The drawing under review shows one solid part. Ordinate dimensions are in mm from its lowest x, y, z. A direction names the side the tool comes from. Round coordinates to 2 decimals unless told otherwise and drop trailing zeros. Loops run counter-clockwise (first coordinate to the right, second up) from the corner with the lowest first, then second, coordinate; pieces in that order, holes last. Notation, with made-up numbers: (61, 44.5) - (91, 44.5) arc R16 ccw to (91, 67.5) - close; hole circle Ø11 at (-38, 11). An arc over 180 degrees is marked (long way). Answer as CSV lines item,"result".
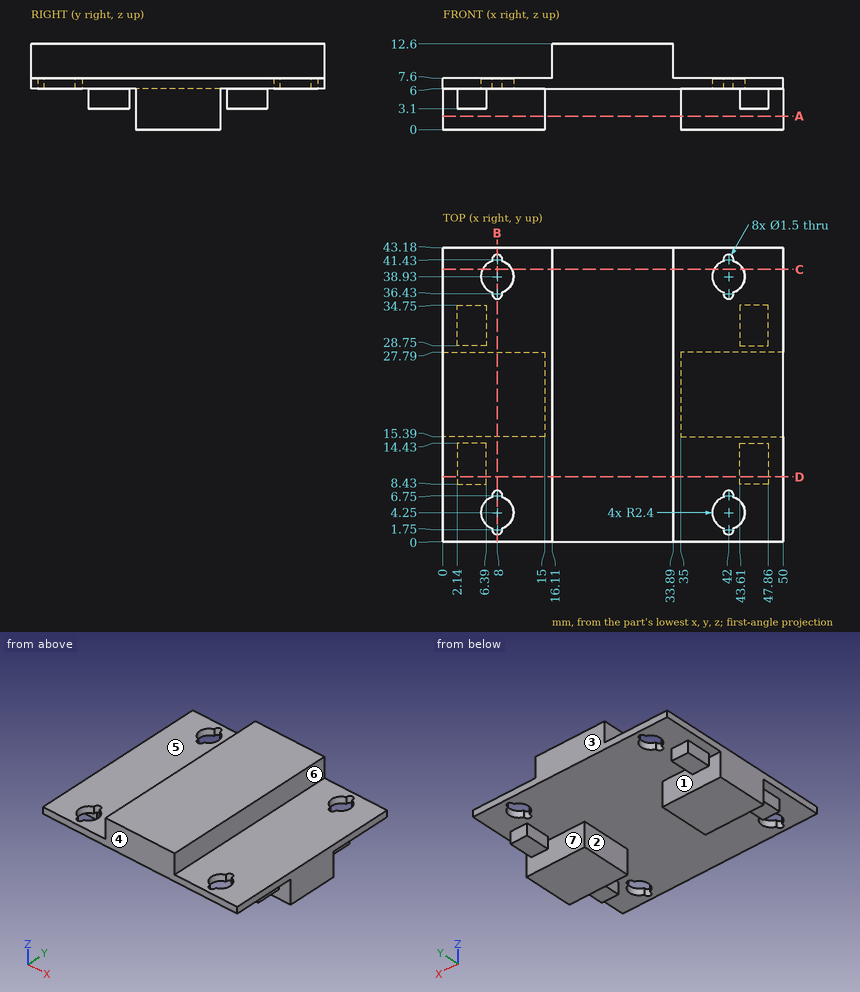
1. Take a section at B-B (x = 8). State the section outline as (y, z) points, plus the area to 3 significant figures.
Numbers:
outline,"(0, 6) - (1, 6) - (1, 7.6) - (0, 7.6) - close; (7.5, 6) - (15.39, 6) - (15.39, 0) - (27.79, 0) - (27.79, 6) - (35.68, 6) - (35.68, 7.6) - (7.5, 7.6) - close; (42.18, 6) - (43.18, 6) - (43.18, 7.6) - (42.18, 7.6) - close"
area,"123 mm²"
2. Wall thickness on probe 1 along X at (y, z) = (6.75, 6.5); probe 2 along X at (y, z) = (23, 3.5); probe 3 along Z at (x, y) = (17.5, 36.5): over which ranges is each line inside the solid? List them lowest first.
Numbers:
probe 1,"x = 0 to 7.25, 8.75 to 41.25, 42.75 to 50"
probe 2,"x = 0 to 15, 35 to 50"
probe 3,"z = 6 to 12.6"
3. Clearance check with flat-ended pins moving along their axes: pin 1 (0.9 mm diameter, centred on y = 32, z = 4.5, fed in from -X); pin 2 (4.5 mm diameter, centred on x = 45, y = 32, fed in from -Z); pin 3 (8 mm diameter, centred on x = 34.5, y = 8.5, fed in from -Z); pin 4 (3 mm diameter, centred on x = 29, z = 5.5, fed in from -Y). State where each tip first meets the part, or that it passes through.
Numbers:
pin 1,"stops at x = 2.14"
pin 2,"stops at z = 3.1"
pin 3,"stops at z = 6"
pin 4,"stops at y = 0"
4. Draft analysis for pull direction Y (two halves, no side actions). For the marked faces 1, 2, 3 and 4, state which applies: +Y half, -Y half, draft (parallel to the pull), parting line (faces both ways), or undercut.
Numbers:
face 1,"undercut"
face 2,"draft"
face 3,"+Y half"
face 4,"-Y half"
5. Take a section at C-C (y = 40). State the section outline as (x, z) points, plus the area to 3 significant figures.
Numbers:
outline,"(0, 6) - (5.85, 6) - (5.85, 7.6) - (0, 7.6) - close; (10.15, 6) - (39.85, 6) - (39.85, 7.6) - (33.89, 7.6) - (33.89, 12.6) - (16.11, 12.6) - (16.11, 7.6) - (10.15, 7.6) - close; (44.15, 6) - (50, 6) - (50, 7.6) - (44.15, 7.6) - close"
area,"155 mm²"
6. Take a section at D-D (y = 9.5). State the section outline as (x, z) points, plus the area to 3 significant figures.
Numbers:
outline,"(0, 6) - (2.14, 6) - (2.14, 3.1) - (6.39, 3.1) - (6.39, 6) - (43.61, 6) - (43.61, 3.1) - (47.86, 3.1) - (47.86, 6) - (50, 6) - (50, 7.6) - (33.89, 7.6) - (33.89, 12.6) - (16.11, 12.6) - (16.11, 7.6) - (0, 7.6) - close"
area,"194 mm²"
7. Tool access review of the marked faces 5, 6 and 7: name each direction out of +Z, -Z, +X, -X, +Y, -Y from which nothing blocks a thin tool from reaching the whole face with its end or side.
Numbers:
face 5,"+Z, -X, +Y, -Y"
face 6,"+Z, +X, +Y, -Y"
face 7,"-Z, +X, -X"
8. Take a section at A-A (z = 2). State the section outline as (x, y) points, plus the area to 3 significant figures.
Numbers:
outline,"(0, 15.39) - (15, 15.39) - (15, 27.79) - (0, 27.79) - close; (35, 15.39) - (50, 15.39) - (50, 27.79) - (35, 27.79) - close"
area,"372 mm²"
